Geometry check sheet. Reference: the model listing, model coordinates, mm. A direction names the side the tool comes from. Give positions to 0.01 mm unless a question says otherwise; leave off trailing zeros. Loops run counter-clockwise (first coordinate to the right, second up) from the corner with the lowest first, then second, coordinate; pieces in that order, holes last.
1. Cross-section at A-A, the plane x = -24. Record the cut outline in (y, z).
2. Go/stop test with flat-tipped pins: pin 1 Ø0.9 at (y, z) = (9, -2.5) entering from -X; pin 2 Ø24 at (x, z) = (-1.5, -3.5) entering from +Y; pin 3 Ø8 at (x, z) = (-22.5, -4.5) entering from +Y. Record where each tip stops, or that it passes through.
3. Cross-section at B-B, the plane z = 0. Record the cut outline in (x, y).
4. Tool access check on faces 5 (the cylindrical face through (-17.57, 8.48, 14.4)), 6 (the cylindrical face through (-2.38, 6.06, 10.74)), 7 (the flat face through (26, 5, -26)). Record the directions out of +Z, -Z, +X, -X, +Y, -Y that give a thin tool (end or side, any length) a straight path to the whole face; none if there is none.
5. Release check for a two-part mould opening along Z. For faces 1 (the flat face through (0, 5, 27)), 2 (the flat face through (6, 0, 6)), 3 (the cylindrical face through (-1.73, 0.99, -7.81)), 4 (the flat face through (-26, 5, -26)) record: +Z half, -Z half, draft (parallel to the pull), parting line (faces both ways), or undercut.
6. Cross-section at D-D, the plane x = 0. Record the cut outline in (y, z).
7. Cross-section at C-C, the plane z = 24. Record the cut outline in (x, y).
8. Material ranges on L1, parallel to Z at x = -24, y = 5.5; L2, parallel to Z at x = 0, y = 0.9, recorded low to high.
Autodesk Inventor part; units mm, degrees
ref_plane "YZ Plane" through (0, 0, 0) normal (1, 0, 0) x (0, 1, 0)
ref_plane "XZ Plane" through (0, 0, 0) normal (0, 1, 0) x (-1, 0, 0)
ref_plane "XY Plane" through (0, 0, 0) normal (0, 0, 1) x (1, 0, 0)
sketch "Skizze1" plane through (0, 0, 0) normal (0, 1, 0) x (-1, 0, 0)
  line L0 (-27, 27) -> (27, 27)
  line L1 (27, 27) -> (27, -27)
  line L2 (27, -27) -> (-27, -27)
  line L3 (-27, -27) -> (-27, 27)
  line L4 (-27, 27) -> (27, -27) construction
  line L5 (27, 27) -> (-27, -27) construction
  point P0 (0, 0)
  dimension "d0" = 54
  dimension "d1" = 54
extrude "Extrusion1" add sketch "Skizze1" along normal blind 10
chamfer "Fase1" distance 2 angle 45 4 edges at (27, 5, 27) (27, 5, -27) (-27, 5, 27) (-27, 5, -27)
sketch "Skizze2" plane through (0, 10, 0) normal (0, 1, 0) x (1, 0, 0)
  circle A0 centre (0, 0) radius 11
  dimension "d7" = 22
extrude "Extrusion2" cut sketch "Skizze2" against normal blind 8
sketch "Skizze5" plane through (0, 0, 0) normal (0, -1, 0) x (1, 0, 0)
  line L0 (-24, -24) -> (24, -24)
  line L1 (24, -24) -> (24, 24)
  line L2 (24, 24) -> (-24, 24)
  line L3 (-24, 24) -> (-24, -24)
  line L4 (-24, -24) -> (24, 24) construction
  line L5 (24, -24) -> (-24, 24) construction
  point P0 (0, 0)
  dimension "d22" = 48
  dimension "d23" = 48
hole "Bohrung2" at (-24, 0, -24) at (-24, 0, 24) at (24, 0, 24) at (24, 0, -24) direction (0, 1, 0) diameter 2.459 end through all
sketch "Skizze6" plane through (0, 0, 0) normal (0, -1, 0) x (1, 0, 0)
  circle A0 centre (0, 0) radius 8
  dimension "d31" = 16
extrude "Extrusion4" cut sketch "Skizze6" against normal through all
sketch "Skizze7" plane through (0, 10, 0) normal (0, 1, 0) x (1, 0, 0)
  circle A0 centre (24, -24) radius 1.2295
  circle A1 centre (-24, 24) radius 1.2295
  circle A2 centre (-24, -24) radius 1.2295
  circle A3 centre (24, 24) radius 1.2295
  circle A4 centre (0, 0) radius 11
  line L0 (-27, 25) -> (-25, 27)
  line L1 (-27, 25) -> (-27, -25)
  line L2 (-25, -27) -> (-27, -25)
  line L3 (-25, -27) -> (25, -27)
  line L4 (27, -25) -> (25, -27)
  line L5 (27, -25) -> (27, 25)
  line L6 (25, 27) -> (27, 25)
  line L7 (25, 27) -> (-25, 27)
  line L8 (-27, -15) -> (-17, -15)
  line L9 (-17, -15) -> (-17, 15)
  line L10 (-17, 15) -> (-27, 15)
  line L11 (-27, 15) -> (-27, -15)
  dimension "d36" = 30
  dimension "d37" = 15
  dimension "d38" = 10
extrude "Extrusion5" cut sketch "Skizze7" against normal blind 3 contours L10 L9 L8 L1
fillet "Rundung1" radius 2 2 edges at (-17, 8.5, 15) (-17, 8.5, -15)
properties part number "bearing_mount_part_2"
Result:
1. outline: (0, -27) - (10, -27) - (10, -25.23) - (0, -25.23) - close; (0, -22.77) - (10, -22.77) - (10, -15) - (7, -15) - (7, 15) - (10, 15) - (10, 22.77) - (0, 22.77) - close; (0, 25.23) - (10, 25.23) - (10, 27) - (0, 27) - close
2. pin 1: stops at x = -17
2. pin 2: stops at y = 10
2. pin 3: stops at y = 7
3. outline: (-27, 0) - (-8, 0) - (-8, 2) - (-11, 2) - (-11, 10) - (-17, 10) - (-17, 7) - (-27, 7) - close; (8, 0) - (27, 0) - (27, 10) - (11, 10) - (11, 2) - (8, 2) - close
4. face 5: -X, +Y
4. face 6: +Y
4. face 7: -Z, +X, +Y, -Y
5. face 1: +Z half
5. face 2: draft
5. face 3: undercut
5. face 4: -Z half
6. outline: (0, -27) - (10, -27) - (10, -11) - (2, -11) - (2, -8) - (0, -8) - close; (0, 8) - (2, 8) - (2, 11) - (10, 11) - (10, 27) - (0, 27) - close
7. outline: (-27, 0) - (-25.23, 0) - (-25.23, 10) - (-27, 10) - close; (-22.77, 0) - (22.77, 0) - (22.77, 10) - (-22.77, 10) - close; (25.23, 0) - (27, 0) - (27, 10) - (25.23, 10) - close
8. L1: z = -27 to -25.23, -22.77 to 22.77, 25.23 to 27
8. L2: z = -27 to -8, 8 to 27
